```python
from build123d import *

# Parameters (mm, degrees)
ESBO_O1_W                     = 12
ESBO_O1_H                     = 20
RESSALTO_EXTRUS_O1_DEPTH      = 14
ESBO_O5_W                     = 12
ESBO_O5_H                     = 10
CORTE_EXTRUS_O1_DEPTH         = 12
RESSALTO_EXTRUS_O2_DEPTH      = 10
RESSALTO_EXTRUS_O2_DEPTH_BACK = 30
ESBO_O6_W                     = 12
ESBO_O6_H                     = 5
ESBO_O7_W                     = 12
ESBO_O7_H                     = 5
CORTE_EXTRUS_O2_DEPTH         = 12
ESBO_O8_R                     = 1.8
CORTE_EXTRUS_O3_DEPTH         = 5
CORTE_EXTRUS_O4_DEPTH         = 5
ESBO_O8_4_R                   = 1.8
CORTE_EXTRUS_O5_DEPTH         = 2.8


with BuildPart() as part:
    # Esbo_o1 → Ressalto-extrus_o1 (new body)
    with BuildSketch(Plane(origin=(0, 0, 0), x_dir=(1, 0, 0), z_dir=(0, 1, 0))):
        Rectangle(ESBO_O1_W, ESBO_O1_H)
    extrude(amount=RESSALTO_EXTRUS_O1_DEPTH)

    # Esbo_o5 → Corte-extrus_o1 (cut)
    with BuildSketch(Plane(origin=(6, 0, 0), x_dir=(0, 0, -1), z_dir=(1, 0, 0))):
        with Locations((0, 5)):
            Rectangle(ESBO_O5_W, ESBO_O5_H)
    extrude(amount=-CORTE_EXTRUS_O1_DEPTH, mode=Mode.SUBTRACT)

    # Esbo_o6 → Ressalto-extrus_o2 (add, two sides: drawn at the far end of the back side and taken through both)
    with BuildSketch(Plane.XY.offset(10).offset(-RESSALTO_EXTRUS_O2_DEPTH_BACK)):
        with Locations((0, 2.5)):
            Rectangle(ESBO_O6_W, ESBO_O6_H)
    extrude(amount=RESSALTO_EXTRUS_O2_DEPTH + RESSALTO_EXTRUS_O2_DEPTH_BACK)

    # Esbo_o7 → Corte-extrus_o2 (cut)
    with BuildSketch(Plane(origin=(6, 0, 0), x_dir=(0, 0, -1), z_dir=(1, 0, 0))):
        with Locations((0, 2.5)):
            Rectangle(ESBO_O7_W, ESBO_O7_H)
    extrude(amount=-CORTE_EXTRUS_O2_DEPTH, mode=Mode.SUBTRACT)

    # Esbo_o8 → Corte-extrus_o3 (cut)
    with BuildSketch(Plane(origin=(0, 5, 0), x_dir=(1, 0, 0), z_dir=(0, 1, 0))):
        with Locations(Location((0.073596401, 14.872527995, 0), (0, 0, 180))):
            Circle(ESBO_O8_R)
    extrude(amount=-CORTE_EXTRUS_O3_DEPTH, mode=Mode.SUBTRACT)

    # Esbo_o8_3 → Corte-extrus_o4 (cut)
    with BuildSketch(Plane(origin=(0, 5, 0), x_dir=(1, 0, 0), z_dir=(0, 1, 0))):
        with BuildLine():
            ThreePointArc((0.973596401, -13.313682268), (-1.485249326, -13.972527995), (-0.826403599, -16.431373721))
            Line((-0.826403599, -16.431373721), (0.973596401, -13.313682268))
        make_face()
        with BuildLine():
            Line((0.973596401, -13.313682268), (-0.826403599, -16.431373721))
            ThreePointArc((-0.826403599, -16.431373721), (0.973596401, -16.431373721), (1.873596401, -14.872527995))
            ThreePointArc((1.873596401, -14.872527995), (1.632442128, -13.972527995), (0.973596401, -13.313682268))
        make_face()
    extrude(amount=-CORTE_EXTRUS_O4_DEPTH, mode=Mode.SUBTRACT)

    # Esbo_o8_4 → Corte-extrus_o5 (cut)
    with BuildSketch(Plane(origin=(0, 5, 0), x_dir=(1, 0, 0), z_dir=(0, 1, 0))):
        with Locations(Location((0.073596401, 14.872527995, 0), (0, 0, 180))):
            Circle(ESBO_O8_4_R)
        Polygon((-1.626403599, 17.817014367), (1.773596401, 11.928041622), (3.473596401, 14.872527995), (1.773596401, 17.817014367), align=None)
        Polygon((-1.626403599, 17.817014367), (1.773596401, 11.928041622), (-1.626403599, 11.928041622), (-3.326403599, 14.872527995), align=None)
        with Locations(Location((0.073596401, -14.872527995, 0), (0, 0, 180))):
            Circle(ESBO_O8_4_R)
        Polygon((-1.626403599, -17.817014367), (1.773596401, -11.928041622), (-1.626403599, -11.928041622), (-3.326403599, -14.872527995), align=None)
        Polygon((-1.626403599, -17.817014367), (1.773596401, -11.928041622), (3.473596401, -14.872527995), (1.773596401, -17.817014367), align=None)
    extrude(amount=-CORTE_EXTRUS_O5_DEPTH, mode=Mode.SUBTRACT)


solid = part.part
```
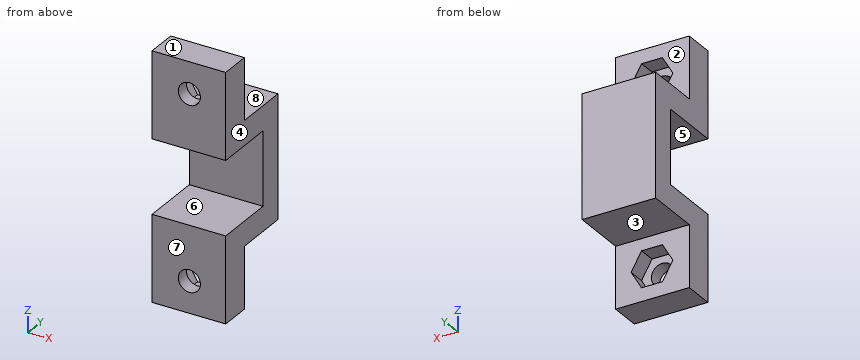
Input: part model. Units: mm. Frame: model coordinates. Face numbers are marked on the shaded views. A direction names the side the tool comes from. Give positions to 0.01 mm unless a question says otherwise; leave off trailing zeros. Order: outer loops, then holes, each group sorted by start corner. A loop starts at its lowest first (then second) coordinate and runs counter-clockwise, first axis right, second up. Notation, with made-up numbers: (10, -38) - (45, -38) arc R18 ccw to (45, -5) - close; hole circle Ø11 at (16, 45.25). An arc over 180 degrees is marked (long way). Use a Markdown table: item, result.
(1) Section query B-B (x = 0.25). Output: boundary loops of the cut face in (y, z), then the cut area to 3 significant figures.
Computed values:
| item | result |
|---|---|
| outline | (0, -20) - (5, -20) - (5, -17.82) - (2.2, -17.82) - (2.2, -16.66) - (0, -16.66) - close; (0, -13.08) - (2.2, -13.08) - (2.2, -11.93) - (5, -11.93) - (5, -10) - (14, -10) - (14, 10) - (5, 10) - (5, 11.93) - (2.2, 11.93) - (2.2, 13.08) - (0, 13.08) - (0, 6) - (10, 6) - (10, -6) - (0, -6) - close; (0, 16.66) - (2.2, 16.66) - (2.2, 17.82) - (5, 17.82) - (5, 20) - (0, 20) - close |
| area | 211 mm2 |
(2) Line query: line 1 (Z direction, x = 0, y = 2); line 2 (Z direction, x = 4.5, y = 9.5); line 3 (Z direction, x = -1.5, y = 4.75). Output: solid intervals per line, ascending. Write a range as from..to.
Computed values:
| item | result |
|---|---|
| line 1 | z = -20..-16.67, -13.07..-6, 6..13.07, 16.67..20 |
| line 2 | z = -10..-6, 6..10 |
| line 3 | z = -20..-17.82, -11.93..-6, 6..11.93, 17.82..20 |
(3) Section query C-C (x = 2.5). Output: boundary loops of the cut face in (y, z).
Computed values:
| item | result |
|---|---|
| outline | (0, -20) - (5, -20) - (5, -16.56) - (2.2, -16.56) - (2.2, -13.19) - (5, -13.19) - (5, -10) - (14, -10) - (14, 10) - (5, 10) - (5, 13.19) - (2.2, 13.19) - (2.2, 16.56) - (5, 16.56) - (5, 20) - (0, 20) - (0, 6) - (10, 6) - (10, -6) - (0, -6) - close |
(4) Access query for the marked faces 1, 2, 3, 4 and 5. Directions: +Z, -Z, +X, -X, +Y, -Y. A direction counts if a zero-diameter tool reaches every point of the face in a straight line with its end or side. Return the directions, or none.
Computed values:
| item | result |
|---|---|
| face 1 | +Z, +X, -X, +Y, -Y |
| face 2 | +Z, +X, -X, +Y |
| face 3 | -Z, +X, -X, +Y |
| face 4 | +Z, -Z, +X, +Y, -Y |
| face 5 | +X, -X, -Y |
(5) Section query D-D (z = 4.5). Output: boundary loops of the cut face in (x, y).
Computed values:
| item | result |
|---|---|
| outline | (-6, 10) - (6, 10) - (6, 14) - (-6, 14) - close |
(6) Section query A-A (y = 7.25). Output: boundary loops of the cut face in (x, z).
Computed values:
| item | result |
|---|---|
| outline | (-6, -10) - (6, -10) - (6, -6) - (-6, -6) - close; (-6, 6) - (6, 6) - (6, 10) - (-6, 10) - close |
(7) Draft query along Z for the marked faces 6, 7 and 8. Return one class per face: released by +Z, released by -Z, zero draft, split by the parting line, or undercut.
Computed values:
| item | result |
|---|---|
| face 6 | undercut |
| face 7 | zero draft |
| face 8 | released by +Z |
(8) Pin query (flat end, axial travel): pin 1 (5 mm diameter, centred on x = 1.5, z = 16, fed in from +Y); pin 2 (3 mm diameter, centred on y = 2.5, z = 3, fed in from -X); pin 3 (2.5 mm diameter, centred on x = 3, y = 8, fed in from -Z); pin 4 (2 mm diameter, centred on x = -2.5, y = 10, fed in from +Z). Return the tip coordinate at first contact, or that it passes through.
Computed values:
| item | result |
|---|---|
| pin 1 | stops at y = 5 |
| pin 2 | passes through |
| pin 3 | stops at z = -10 |
| pin 4 | stops at z = 10 |
